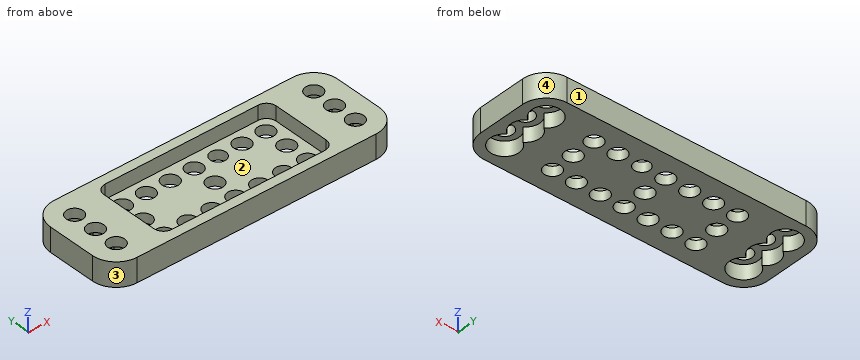
from build123d import *

# Parameters (mm, degrees)
F0_W     = 36
F0_H     = 16
F0_R     = 1.75
F0_R_2   = 1.6342219217
F1_DEPTH = 2
F0_W_2   = 60
F0_H_2   = 20
F2_DEPTH = 3
F3_W     = 60
F3_H     = 20
F3_W_2   = 36
F3_H_2   = 16
F4_DEPTH = 2
F5_DEPTH = 25
F6_R     = 5
F7_R     = 2


with BuildPart() as f1:
    # F0 (on Top) → F1 (new body)
    with BuildSketch(Plane.XY):
        with Locations((-6.9101825356, 29.7833877802)):
            Rectangle(F0_W, F0_H)
        with Locations((-21.9101825356, 24.7833877802)):
            Circle(F0_R, mode=Mode.SUBTRACT)
        with Locations((-16.9101825356, 24.7833877802)):
            Circle(F0_R, mode=Mode.SUBTRACT)
        with Locations((-11.9101825356, 24.7833877802)):
            Circle(F0_R, mode=Mode.SUBTRACT)
        with Locations((-6.9101825356, 24.7833877802)):
            Circle(F0_R, mode=Mode.SUBTRACT)
        with Locations((-1.9101825356, 24.7833877802)):
            Circle(F0_R, mode=Mode.SUBTRACT)
        with Locations((3.0898174644, 24.7833877802)):
            Circle(F0_R, mode=Mode.SUBTRACT)
        with Locations((8.0898174644, 24.7833877802)):
            Circle(F0_R, mode=Mode.SUBTRACT)
        with Locations((-21.9101825356, 29.7833877802)):
            Circle(F0_R, mode=Mode.SUBTRACT)
        with Locations((-21.9101825356, 34.7833877802)):
            Circle(F0_R, mode=Mode.SUBTRACT)
        with Locations((-16.9101825356, 34.7833877802)):
            Circle(F0_R, mode=Mode.SUBTRACT)
        with Locations((-11.9101825356, 34.7833877802)):
            Circle(F0_R, mode=Mode.SUBTRACT)
        with Locations((-6.9101825356, 29.7833877802)):
            Circle(F0_R, mode=Mode.SUBTRACT)
        with Locations((8.0898174644, 29.7833877802)):
            Circle(F0_R, mode=Mode.SUBTRACT)
        with Locations((-6.9101825356, 34.7833877802)):
            Circle(F0_R, mode=Mode.SUBTRACT)
        with Locations((-1.9101825356, 34.7833877802)):
            Circle(F0_R_2, mode=Mode.SUBTRACT)
        with Locations((3.0898174644, 34.7833877802)):
            Circle(F0_R, mode=Mode.SUBTRACT)
        with Locations((8.0898174644, 34.7833877802)):
            Circle(F0_R, mode=Mode.SUBTRACT)
    extrude(amount=F1_DEPTH)

    # F0 (on Top) → F2 (join)
    with BuildSketch(Plane.XY):
        with Locations((-6.9101825356, 29.7833877802)):
            Rectangle(F0_W_2, F0_H_2)
        with Locations((-6.9101825356, 29.7833877802)):
            Rectangle(F0_W, F0_H, mode=Mode.SUBTRACT)
        with BuildLine():
            ThreePointArc((-30.2518701405, 27.2833877802), (-31.9101825356, 21.7833877802), (-33.5684949308, 27.2833877802))
            ThreePointArc((-33.5684949308, 27.2833877802), (-34.9101825356, 29.7833877802), (-33.5684949308, 32.2833877802))
            ThreePointArc((-33.5684949308, 32.2833877802), (-31.9101825356, 37.7833877802), (-30.2518701405, 32.2833877802))
            ThreePointArc((-30.2518701405, 32.2833877802), (-28.9101825356, 29.7833877802), (-30.2518701405, 27.2833877802))
        make_face(mode=Mode.SUBTRACT)
        with BuildLine():
            ThreePointArc((19.7481298595, 27.2833877802), (18.0898174644, 21.7833877802), (16.4315050692, 27.2833877802))
            ThreePointArc((16.4315050692, 27.2833877802), (15.0898174644, 29.7833877802), (16.4315050692, 32.2833877802))
            ThreePointArc((16.4315050692, 32.2833877802), (18.0898174644, 37.7833877802), (19.7481298595, 32.2833877802))
            ThreePointArc((19.7481298595, 32.2833877802), (21.0898174644, 29.7833877802), (19.7481298595, 27.2833877802))
        make_face(mode=Mode.SUBTRACT)
    extrude(amount=F2_DEPTH)

    # F3 (on face) → F4 (join)
    with BuildSketch(Plane.XY.offset(3)):
        with Locations((-6.9101825356, 29.7833877802)):
            Rectangle(F3_W, F3_H)
        with Locations((-6.9101825356, 29.7833877802)):
            Rectangle(F3_W_2, F3_H_2, mode=Mode.SUBTRACT)
        with BuildLine():
            ThreePointArc((-33.5684949308, 32.2833877802), (-31.9101825356, 37.7833877802), (-30.2518701405, 32.2833877802))
            ThreePointArc((-30.2518701405, 32.2833877802), (-28.9101825356, 29.7833877802), (-30.2518701405, 27.2833877802))
            ThreePointArc((-30.2518701405, 27.2833877802), (-31.9101825356, 21.7833877802), (-33.5684949308, 27.2833877802))
            ThreePointArc((-33.5684949308, 27.2833877802), (-34.9101825356, 29.7833877802), (-33.5684949308, 32.2833877802))
        make_face(mode=Mode.SUBTRACT)
        with BuildLine():
            ThreePointArc((16.4315050692, 32.2833877802), (18.0898174644, 37.7833877802), (19.7481298595, 32.2833877802))
            ThreePointArc((19.7481298595, 32.2833877802), (21.0898174644, 29.7833877802), (19.7481298595, 27.2833877802))
            ThreePointArc((19.7481298595, 27.2833877802), (18.0898174644, 21.7833877802), (16.4315050692, 27.2833877802))
            ThreePointArc((16.4315050692, 27.2833877802), (15.0898174644, 29.7833877802), (16.4315050692, 32.2833877802))
        make_face(mode=Mode.SUBTRACT)
        with BuildLine():
            ThreePointArc((19.7481298595, 27.2833877802), (21.0898174644, 29.7833877802), (19.7481298595, 32.2833877802))
            ThreePointArc((19.7481298595, 32.2833877802), (18.0898174644, 37.7833877802), (16.4315050692, 32.2833877802))
            ThreePointArc((16.4315050692, 32.2833877802), (15.0898174644, 29.7833877802), (16.4315050692, 27.2833877802))
            ThreePointArc((16.4315050692, 27.2833877802), (18.0898174644, 21.7833877802), (19.7481298595, 27.2833877802))
        make_face()
        with BuildLine():
            ThreePointArc((-30.2518701405, 27.2833877802), (-28.9101825356, 29.7833877802), (-30.2518701405, 32.2833877802))
            ThreePointArc((-30.2518701405, 32.2833877802), (-31.9101825356, 37.7833877802), (-33.5684949308, 32.2833877802))
            ThreePointArc((-33.5684949308, 32.2833877802), (-34.9101825356, 29.7833877802), (-33.5684949308, 27.2833877802))
            ThreePointArc((-33.5684949308, 27.2833877802), (-31.9101825356, 21.7833877802), (-30.2518701405, 27.2833877802))
        make_face()
    extrude(amount=F4_DEPTH)

    # F0 (on Top) → F5 (cut)
    with BuildSketch(Plane.XY):
        with Locations((-31.9101825356, 34.7833877802)):
            Circle(F0_R)
        with Locations((-31.9101825356, 29.7833877802)):
            Circle(F0_R)
        with Locations((-31.9101825356, 24.7833877802)):
            Circle(F0_R)
        with Locations((18.0898174644, 24.7833877802)):
            Circle(F0_R)
        with Locations((18.0898174644, 34.7833877802)):
            Circle(F0_R)
        with Locations((18.0898174644, 29.7833877802)):
            Circle(F0_R)
    extrude(amount=F5_DEPTH, mode=Mode.SUBTRACT)

    # F6
    f6_edges = [f1.edges().sort_by_distance(p)[0] for p in [
        (-36.910183, 39.783388, 2.5),
        (-36.910183, 19.783388, 2.5),
        (23.089817, 19.783388, 2.5),
        (23.089817, 39.783388, 2.5),
    ]]
    fillet(f6_edges, radius=F6_R)

    # F7
    f7_edges = [f1.edges().sort_by_distance(p)[0] for p in [
        (-24.910183, 37.783388, 3.5),
        (11.089817, 21.783388, 3.5),
        (11.089817, 37.783388, 3.5),
        (-24.910183, 21.783388, 3.5),
    ]]
    fillet(f7_edges, radius=F7_R)


solid = f1.part
Check sheet for the modelled part. Datum: model origin and axes. Units: mm. Face numbers are marked on the shaded views. Give positions to 0.01 mm unless a question says otherwise; leave off trailing zeros. Write each loop counter-clockwise with the first axis right and the second up, starting at its lowest first coordinate (ties: lowest second). Pieces come first, ordered by that corner, then holes. Notation, with made-up numbers: M 84,27 L 101,27 A24 cw 101,56 Z; hole C 85,49.5 d7. An arc over 180 degrees is marked long. Use one line per item in the form item = value.
(1) Section check D-D on x = -29.5. Record the boundary of the cut face in (y, z), plus the area to 3 significant figures.
Answer block:
outline = M 19.78,0 L 23,0 L 23,3 L 26.57,3 L 26.57,0 L 28,0 L 28,3 L 31.57,3 L 31.57,0 L 33,0 L 33,3 L 36.57,3 L 36.57,0 L 39.78,0 L 39.78,5 L 19.78,5 Z
area = 67.8 mm2
(2) Material ranges on line 1 along X through (y, z) = (29.5, 2.5); line 2 along Y through (x, z) = (-11, 2.75); line 3 along X through (y, z) = (27.5, 3.55), recorded low to high.
Answer block:
line_1 = -36.91 to -34.9, -28.92 to -24.91, 11.09 to 15.1, 21.08 to 23.09
line_2 = 19.78 to 21.78, 37.78 to 39.78
line_3 = -36.91 to -24.91, 11.09 to 23.09
(3) Section check A-A on z = 1.05. State how many separate pieces and enclosed holes the cut face has, plus the area to 3 significant figures.
Answer block:
separate_pieces = 1
enclosed_holes = 19
area = 856 mm2
(4) Section check C-C on z = 3.75. Record the boundary of the cut face in (x, y).
Answer block:
outline = M -36.91,24.78 A5 ccw -31.91,19.78 L 18.09,19.78 A5 ccw 23.09,24.78 L 23.09,34.78 A5 ccw 18.09,39.78 L -31.91,39.78 A5 ccw -36.91,34.78 Z; hole C -31.91,24.78 d3.5; hole C -31.91,29.78 d3.5; hole C -31.91,34.78 d3.5; hole M -24.91,23.78 A2 ccw -22.91,21.78 L 9.09,21.78 A2 ccw 11.09,23.78 L 11.09,35.78 A2 ccw 9.09,37.78 L -22.91,37.78 A2 ccw -24.91,35.78 Z; hole C 18.09,24.78 d3.5; hole C 18.09,29.78 d3.5; hole C 18.09,34.78 d3.5
(5) Draft check along X on the marked faces 1, 2, 3 and 4. Enter one of: pulls with the +X half, pulls with the -X half, needs draft (parallel to the pull), parting line crosses it, or undercut.
Answer block:
face_1 = needs draft
face_2 = undercut
face_3 = pulls with the -X half
face_4 = pulls with the +X half
(6) Section check B-B on x = -12. Record the boundary of the cut face in (y, z).
Answer block:
outline = M 19.78,0 L 23.04,0 L 23.04,2 L 21.78,2 L 21.78,5 L 19.78,5 Z; M 26.53,0 L 33.04,0 L 33.04,2 L 26.53,2 Z; M 36.53,0 L 39.78,0 L 39.78,5 L 37.78,5 L 37.78,2 L 36.53,2 Z
(7) Depth check by flat-ended pin: P1, Ø3, axis at x = 8.09, y = 34.78, coming from the +Z side; P2, Ø5.5, axis at x = -21.91, y = 24.78, coming from the +Z side. Enter the tip coordinate at first touch or a pass-through.
Answer block:
P1 = through
P2 = 2
